```python
from build123d import *

# Parameters (mm, degrees)
CROQUIS2_R = 6.35
CROQUIS7_R = 6.35
CROQUIS8_R = 6.35


with BuildPart() as part:
    # Barrer2: sweep along a path in Croquis1
    with BuildLine(Plane(origin=(0, 0, 0), x_dir=(1, 0, 0), z_dir=(0, 1, 0))) as barrer2_path:
        Line((0, 0), (50, 0))
        ThreePointArc((50, 0), (64.142135624, -5.857864376), (70, -20))
        Line((70, -20), (70, -70))
    # Croquis2 → Barrer2 (sweep)
    with BuildSketch(Plane(origin=(0, 0, 0), x_dir=(0, 0, -1), z_dir=(1, 0, 0))):
        Circle(CROQUIS2_R)
    sweep(path=barrer2_path.line)

    # Barrer3: sweep along a path in Croquis3
    with BuildLine(Plane(origin=(70, 0, 0), x_dir=(0, 0, -1), z_dir=(1, 0, 0))) as barrer3_path:
        Line((-70, 0), (-99.387787897, 0))
        ThreePointArc((-99.387787897, 0), (-113.529923521, -5.857864376), (-119.387787897, -20))
        Line((-119.387787897, -20), (-119.387787897, -40.166140684))
        Line((-119.387787897, -40.166140684), (-119.387787897, -49.955998728))
    # Croquis7 → Barrer3 (sweep)
    with BuildSketch(Plane.XY.offset(70)):
        with Locations((70, 0)):
            Circle(CROQUIS7_R)
    sweep(path=barrer3_path.line)

    # Barrer4: sweep along a path in Croquis5
    with BuildLine(Plane.XY.offset(119.387787897)) as barrer4_path:
        Line((70, -49.842890924), (70, -66.211244979))
        ThreePointArc((70, -66.211244979), (75.857864376, -80.353380602), (90, -86.211244979))
        Line((90, -86.211244979), (126.42207306, -86.211244979))
    # Croquis8 → Barrer4 (sweep)
    with BuildSketch(Plane.XZ.offset(49.955998728)):
        with Locations((70, 119.387787897)):
            Circle(CROQUIS8_R)
    sweep(path=barrer4_path.line)


solid = part.part
```
Input: part model. Units: mm. Frame: model coordinates. A direction names the side the tool comes from. Coordinates: 2 decimals unless noted, no trailing zeros. Loops run counter-clockwise (first coordinate to the right, second up) from the corner with the lowest first, then second, coordinate; pieces in that order, holes last. Notation, with made-up numbers: M 24,-6 L 79,-6 A18 ccw 79,5 Z; hole C 58.5,-12.75 d8. An arc over 180 degrees is marked long. Use a Markdown table: item, result. Add a question column.
1) Pin query (flat end, axial travel): P1, Ø10, axis at y = -13, z = 103.5, coming from the -X side; P2, Ø12, axis at x = 27.5, y = -8, coming from the +Z side. Return the tip coordinate at first contact, or that it passes through.
2) Set-up query: faces 1 (the cylindrical face through (108.466, -91.25, 115.524)), 2 (the flat face through (126.422, -86, 119)), 3 (the cylindrical face through (25.35, -6.2, 1.38)). Return all of +Z, -Z, +X, -X, +Y, -Y with unobstructed straight access to the full face (end or side cutting, diameter ignored); none if empty.
3) Draft query along Z for faces 4 (the cylindrical face through (76.057, 1.907, 60.25)), 5 (the flat face through (0, 0, 0)), 6 (the cylindrical face through (72.93, -43.429, 113.754)). Return one class per face: +Z half, -Z half, draft (parallel to the pull), parting line (faces both ways), or undercut.
4) Section A-A, the plane z = 79. Return the cut outline in (x, y), plus the area to 3 significant figures.
5) Section B-B, the plane y = -37. Return the cut outline in (x, z), plus the area to 3 significant figures.
6) Line query: L1, parallel to Z at x = 98, y = -83; L2, parallel to Y at x = 65.5, z = 0.5; L3, parallel to Y at x = 82.5, z = 117. Output: solid intervals per line, ascending. Write a range as from..to.
Answer below:
| question | item | result |
|---|---|---|
| 1 | P1 | through |
| 1 | P2 | z = 6.03 |
| 2 | face 1 | +X |
| 2 | face 2 | +Z, -Z, +X, +Y, -Y |
| 2 | face 3 | -X |
| 3 | face 4 | undercut |
| 3 | face 5 | draft |
| 3 | face 6 | parting line |
| 4 | outline | C 70,0 d12.7 |
| 4 | area | 127 mm2 |
| 5 | outline | C 70,119.39 d12.7 |
| 5 | area | 127 mm2 |
| 6 | L1 | 113.91..124.87 |
| 6 | L2 | -4.03..4.03 |
| 6 | L3 | -90.98..-78.17 |
